The model under review builds one solid part; all positions refer to its coordinate system, in mm. Round coordinates to 2 decimals unless told otherwise and drop trailing zeros. Write each loop counter-clockwise with the first axis right and the second up, starting at its lowest first coordinate (ties: lowest second). Pieces come first, ordered by that corner, then holes. Notation, with made-up numbers: (50, 80) - (84, 80) arc R19 cw to (84, 110) - close; hole circle Ø7 at (-26.5, 31.25). An arc over 180 degrees is marked (long way). Write each question's results on one line, items separated by ' | '.
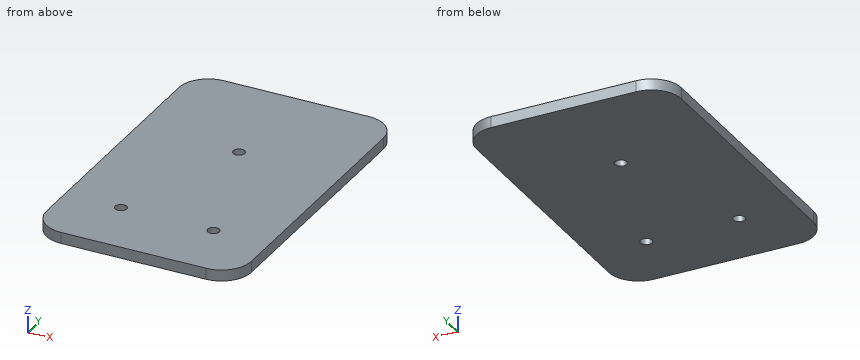
```python
from build123d import *

# Parameters (mm, degrees)
F0_W     = 55
F0_H     = 85
F1_DEPTH = 3
F2_R     = 1.55
F3_DEPTH = 3
F4_R     = 8


with BuildPart() as f1:
    # F0 (on Top) → F1 (new body)
    with BuildSketch(Plane.XY):
        Rectangle(F0_W, F0_H)
    extrude(amount=F1_DEPTH)

    # F2 (on face) → F3 (cut, through all)
    with BuildSketch(Plane.XY.offset(3)):
        with Locations((-12.45, -24.95)):
            Circle(F2_R)
        with Locations((12.45, -24.95)):
            Circle(F2_R)
        with Locations((0, 12.55)):
            Circle(F2_R)
    extrude(amount=-F3_DEPTH, mode=Mode.SUBTRACT)

    # F4
    f4_edges = [f1.edges().sort_by_distance(p)[0] for p in [
        (27.5, -42.5, 1.5),
        (-27.5, -42.5, 1.5),
        (-27.5, 42.5, 1.5),
        (27.5, 42.5, 1.5),
    ]]
    fillet(f4_edges, radius=F4_R)


solid = f1.part
```
Q1. We need section A-A (y = 12.55). State the section outline as (x, z) points, plus the area to 3 significant figures.
Evaluation:
outline: (-27.5, 0) - (-1.55, 0) - (-1.55, 3) - (-27.5, 3) - close; (1.55, 0) - (27.5, 0) - (27.5, 3) - (1.55, 3) - close | area: 156 mm^2
Q2. We need section D-D (z = 1.75). State the section outline as (x, y) points, plus the area to 3 significant figures.
Evaluation:
outline: (-27.5, -34.5) arc R8 ccw to (-19.5, -42.5) - (19.5, -42.5) arc R8 ccw to (27.5, -34.5) - (27.5, 34.5) arc R8 ccw to (19.5, 42.5) - (-19.5, 42.5) arc R8 ccw to (-27.5, 34.5) - close; hole circle Ø3.1 at (-12.45, -24.95); hole circle Ø3.1 at (0, 12.55); hole circle Ø3.1 at (12.45, -24.95) | area: 4,600 mm^2
Q3. We need section B-B (x = 12.45). State the section outline as (y, z) points, plus the area to 3 significant figures.
Evaluation:
outline: (-42.5, 0) - (-26.5, 0) - (-26.5, 3) - (-42.5, 3) - close; (-23.4, 0) - (42.5, 0) - (42.5, 3) - (-23.4, 3) - close | area: 246 mm^2
Q4. We need section C-C (y = -24.95). State the section outline as (x, z) points.
Evaluation:
outline: (-27.5, 0) - (-14, 0) - (-14, 3) - (-27.5, 3) - close; (-10.9, 0) - (10.9, 0) - (10.9, 3) - (-10.9, 3) - close; (14, 0) - (27.5, 0) - (27.5, 3) - (14, 3) - close
Q5. For probe 1 along Y at (x, z) = (0, 1.65); probe 2 along Y at (x, z) = (-12.45, 1.75); probe 3 along X at (y, z) = (39, 1.8), list the stretches that pass through material, from the lowest coordinate up.
Evaluation:
probe 1: y = -42.5 to 11, 14.1 to 42.5 | probe 2: y = -42.5 to -26.5, -23.4 to 42.5 | probe 3: x = -26.11 to 26.11
Q6. Insertion check: P1, Ø3, axis at x = -12.45, y = -24.95, coming from the +Z side. The pin has a flat end and moves straight along its axis. Give the tip position at first contact, or say it passes through.
Evaluation:
P1: passes through
